```python
from build123d import *

# Parameters (mm, degrees)
BOSS_EXTRUDE1_DEPTH          = 90
SKETCH2_R                    = 7.55
SKETCH2_R_2                  = 5.5
CUT_EXTRUDE1_DEPTH           = 90
SKETCH3_R                    = 4.075
CUT_EXTRUDE2_DEPTH           = 90
CUT_EXTRUDE3_START           = -42
SKETCH4_W                    = 84
SKETCH4_H                    = 50
SKETCH4_R                    = 4.075
CUT_EXTRUDE3_DEPTH           = 42
SKETCH5_R                    = 11.5
SKETCH5_R_2                  = 1.75
CUT_EXTRUDE4_DEPTH           = 42
SKETCH10_W                   = 1
SKETCH10_H                   = 23.85052841
CUT_EXTRUDE_THIN1_DEPTH      = 70
CHAMFER2_SIZE                = 2
BOSS_EXTRUDE4_DEPTH          = 3
SKETCH15_W                   = 15
SKETCH15_H                   = 60
BOSS_EXTRUDE5_DEPTH          = 3
FILLET1_R                    = 5
SKETCH16_W                   = 84
SKETCH16_H                   = 42
CUT_EXTRUDE5_DEPTH           = 10
BOSS_EXTRUDE6_DEPTH          = 84
BOSS_EXTRUDE7_START          = -9
SKETCH18_R                   = 4.075
BOSS_EXTRUDE7_DEPTH          = 9
CUT_EXTRUDE_THIN3_DEPTH      = 121.933866311
CUT_EXTRUDE_THIN3_DEPTH_BACK = 9
SKETCH21_R                   = 11.5
CUT_EXTRUDE7_DEPTH           = 7
SKETCH22_R                   = 1.95
CUT_EXTRUDE8_DEPTH           = 20
SKETCH23_W                   = 15
SKETCH23_H                   = 5
CUT_EXTRUDE9_DEPTH           = 20
BOSS_EXTRUDE8_REACH          = 103.367
CHAMFER3_SIZE                = 5
CHAMFER4_SIZE                = 5


with BuildPart() as part:
    # Sketch1 → Boss-Extrude1 (new body)
    with BuildSketch(Plane(origin=(0, 0, 0), x_dir=(0, 0, -1), z_dir=(1, 0, 0))):
        with BuildLine():
            Line((-27.5, -30), (27.5, -30))
            ThreePointArc((27.5, -30), (31.035533906, -28.535533906), (32.5, -25))
            Line((32.5, -25), (32.5, 25))
            ThreePointArc((32.5, 25), (31.035533906, 28.535533906), (27.5, 30))
            Line((27.5, 30), (-27.5, 30))
            ThreePointArc((-27.5, 30), (-31.035533906, 28.535533906), (-32.5, 25))
            Line((-32.5, 25), (-32.5, -25))
            ThreePointArc((-32.5, -25), (-31.035533906, -28.535533906), (-27.5, -30))
        make_face()
    extrude(amount=BOSS_EXTRUDE1_DEPTH)

    # Sketch2 → Cut-Extrude1 (cut)
    with BuildSketch(Plane(origin=(0, 30, 0), x_dir=(1, 0, 0), z_dir=(0, 1, 0))):
        with Locations(Location((10, -18.5, 0), (0, 0, 270))):
            Circle(SKETCH2_R)
        with Locations(Location((80, -18.5, 0), (0, 0, 270))):
            Circle(SKETCH2_R)
        with Locations(Location((45, -18.5, 0), (0, 0, 270))):
            Circle(SKETCH2_R_2)
    extrude(amount=-CUT_EXTRUDE1_DEPTH, mode=Mode.SUBTRACT)

    # Sketch3 → Cut-Extrude2 (cut)
    with BuildSketch(Plane.XY.offset(32.5)):
        with Locations((20, 0)):
            Circle(SKETCH3_R)
        with Locations((70, 0)):
            Circle(SKETCH3_R)
    extrude(amount=-CUT_EXTRUDE2_DEPTH, mode=Mode.SUBTRACT)

    # Sketch4 → Cut-Extrude3 (cut)
    with BuildSketch(Plane(origin=(0, 0, -32.5), x_dir=(-1, 0, 0), z_dir=(0, 0, -1)).offset(CUT_EXTRUDE3_START)):
        with Locations((-45, 0)):
            Rectangle(SKETCH4_W, SKETCH4_H)
        with Locations(Location((-70, 0, 0), (0, 0, 180))):
            Circle(SKETCH4_R, mode=Mode.SUBTRACT)
        with Locations(Location((-20, 0, 0), (0, 0, 180))):
            Circle(SKETCH4_R, mode=Mode.SUBTRACT)
    extrude(amount=CUT_EXTRUDE3_DEPTH, mode=Mode.SUBTRACT)

    # Sketch5 → Cut-Extrude4 (cut)
    with BuildSketch(Plane(origin=(3, 0, 0), x_dir=(0, 0, -1), z_dir=(1, 0, 0))):
        with Locations((12, 0)):
            Circle(SKETCH5_R)
        with Locations((-3.5, 15.5)):
            Circle(SKETCH5_R_2)
        with Locations((27.5, 15.5)):
            Circle(SKETCH5_R_2)
        with Locations((27.5, -15.5)):
            Circle(SKETCH5_R_2)
        with Locations((-3.5, -15.5)):
            Circle(SKETCH5_R_2)
    extrude(amount=-CUT_EXTRUDE4_DEPTH, mode=Mode.SUBTRACT)

    # Sketch10 → Cut-Extrude-Thin1 (cut)
    with BuildSketch(Plane(origin=(0, 30, 0), x_dir=(1, 0, 0), z_dir=(0, 1, 0))):
        with Locations((10, -30.425264205)):
            Rectangle(SKETCH10_W, SKETCH10_H)
        with Locations((80, -30.425264205)):
            Rectangle(SKETCH10_W, SKETCH10_H)
    extrude(amount=-CUT_EXTRUDE_THIN1_DEPTH, mode=Mode.SUBTRACT)

    # Chamfer2
    chamfer2_edges = [part.edges().sort_by_distance(p)[0] for p in [
        (3, 0, -0.5),
    ]]
    chamfer(chamfer2_edges, length=CHAMFER2_SIZE)

    # Sketch14 → Boss-Extrude4 (add)
    with BuildSketch(Plane.ZY):
        with BuildLine():
            Line((-27.5, -30), (-42.5, -30))
            Line((-42.5, -30), (-42.5, 30))
            Line((-42.5, 30), (-27.5, 30))
            ThreePointArc((-27.5, 30), (-31.035533906, 28.535533906), (-32.5, 25))
            Line((-32.5, 25), (-32.5, -25))
            ThreePointArc((-32.5, -25), (-31.035533906, -28.535533906), (-27.5, -30))
        make_face()
    extrude(amount=-BOSS_EXTRUDE4_DEPTH)

    # Sketch15 → Boss-Extrude5 (add)
    with BuildSketch(Plane(origin=(90, 0, 0), x_dir=(0, 0, -1), z_dir=(1, 0, 0))):
        with Locations((35, 0)):
            Rectangle(SKETCH15_W, SKETCH15_H)
    extrude(amount=-BOSS_EXTRUDE5_DEPTH)

    # Fillet1
    fillet1_edges = [part.edges().sort_by_distance(p)[0] for p in [
        (1.5, -30, -42.5),
        (1.5, 30, -42.5),
        (88.5, 30, -42.5),
        (88.5, -30, -42.5),
    ]]
    fillet(fillet1_edges, radius=FILLET1_R)

    # Sketch16 → Cut-Extrude5 (cut)
    with BuildSketch(Plane(origin=(0, -25, 0), x_dir=(1, 0, 0), z_dir=(0, 1, 0))):
        with Locations((45, 11.5)):
            Rectangle(SKETCH16_W, SKETCH16_H)
    extrude(amount=-CUT_EXTRUDE5_DEPTH, mode=Mode.SUBTRACT)

    # Sketch17 → Boss-Extrude6 (add)
    with BuildSketch(Plane(origin=(3, 0, 0), x_dir=(0, 0, -1), z_dir=(1, 0, 0))):
        with BuildLine():
            Line((32.5, 25), (42.5, 25))
            ThreePointArc((42.5, 25), (41.035533906, 28.535533906), (37.5, 30))
            Line((37.5, 30), (27.5, 30))
            ThreePointArc((27.5, 30), (31.035533906, 28.535533906), (32.5, 25))
        make_face()
    extrude(amount=BOSS_EXTRUDE6_DEPTH)

    # Sketch18 → Boss-Extrude7 (add)
    with BuildSketch(Plane(origin=(0, 0, -42.5), x_dir=(-1, 0, 0), z_dir=(0, 0, -1)).offset(BOSS_EXTRUDE7_START)):
        with BuildLine():
            Line((-61, 0), (-61, 25))
            Line((-61, 25), (-87, 25))
            Line((-87, 25), (-87, -9))
            Line((-87, -9), (-70, -9))
            ThreePointArc((-70, -9), (-63.636038969, -6.363961031), (-61, 0))
        make_face()
        with Locations(Location((-70, 0, 0), (0, 0, 180))):
            Circle(SKETCH18_R, mode=Mode.SUBTRACT)
    extrude(amount=BOSS_EXTRUDE7_DEPTH)

    # Sketch19 → Cut-Extrude-Thin3 (cut, two sides: drawn at the far end of the back side and taken through both)
    with BuildSketch(Plane(origin=(0, 0, -42.5), x_dir=(-1, 0, 0), z_dir=(0, 0, -1)).offset(-CUT_EXTRUDE_THIN3_DEPTH_BACK)):
        Polygon((-61.965111244, -7.327781975), (-63.282485579, -6.01040764), (-66.764986476, -2.527906743), (-68.355005201, -0.937888018), (-69.062111982, -1.644994799), (-67.472093257, -3.235013524), (-63.98959236, -6.717514421), (-62.672218025, -8.034888756), align=None)
    extrude(amount=CUT_EXTRUDE_THIN3_DEPTH + CUT_EXTRUDE_THIN3_DEPTH_BACK, mode=Mode.SUBTRACT)

    # Sketch21 → Cut-Extrude7 (cut)
    with BuildSketch(Plane(origin=(0, 30, 0), x_dir=(1, 0, 0), z_dir=(0, 1, 0))):
        with Locations(Location((45, -18.5, 0), (0, 0, 231.500049591))):
            Circle(SKETCH21_R)
    extrude(amount=-CUT_EXTRUDE7_DEPTH, mode=Mode.SUBTRACT)

    # Sketch22 → Cut-Extrude8 (cut)
    with BuildSketch(Plane(origin=(0, 23, 0), x_dir=(1, 0, 0), z_dir=(0, 1, 0))):
        with Locations(Location((53, -18.5, 0), (0, 0, 270))):
            Circle(SKETCH22_R)
        with Locations(Location((45, -26.5, 0), (0, 0, 270))):
            Circle(SKETCH22_R)
        with Locations(Location((37, -18.5, 0), (0, 0, 270))):
            Circle(SKETCH22_R)
    extrude(amount=-CUT_EXTRUDE8_DEPTH, mode=Mode.SUBTRACT)

    # Sketch23 → Cut-Extrude9 (cut)
    with BuildSketch(Plane(origin=(3, 0, 0), x_dir=(0, 0, -1), z_dir=(1, 0, 0))):
        with Locations((12, 22.5)):
            Rectangle(SKETCH23_W, SKETCH23_H)
    extrude(amount=-CUT_EXTRUDE9_DEPTH, mode=Mode.SUBTRACT)

    # Sketch24 → Boss-Extrude8 (add, up to next)
    with BuildSketch(Plane.ZY.offset(-87), mode=Mode.PRIVATE) as boss_extrude8_sk1:
        with BuildLine():
            Line((-42.5, -21), (-33.5, -21))
            Line((-33.5, -21), (-33.5, -30))
            Line((-33.5, -30), (-37.5, -30))
            ThreePointArc((-37.5, -30), (-41.035533906, -28.535533906), (-42.5, -25))
            Line((-42.5, -25), (-42.5, -21))
        make_face()
    boss_extrude8_tool1 = extrude(boss_extrude8_sk1.sketch, amount=BOSS_EXTRUDE8_REACH, mode=Mode.PRIVATE) - part.part
    add(boss_extrude8_tool1.solids().sort_by_distance((87, -25.260021, -37.760021))[0])

    # Chamfer3
    chamfer3_edges = [part.edges().sort_by_distance(p)[0] for p in [
        (87, -9, -38),
        (3, -21, -38),
        (87, -21, -38),
    ]]
    chamfer(chamfer3_edges, length=CHAMFER3_SIZE)

    # Chamfer4
    # the kernel refuses this chamfer: 5 mm, written as the material it adds along each edge
    with BuildSketch(Plane(origin=(61, 25, -33.5), x_dir=(0.027495876610586317, -0.9996219169112968, 0), z_dir=(0, 0, -1))) as chamfer4_piece_1:
        Polygon((CHAMFER4_SIZE * 0.999621916911, CHAMFER4_SIZE * 0.0274958766106), (-CHAMFER4_SIZE * 0.0274958766106, CHAMFER4_SIZE * 0.999621916911), (0, 0), align=None)
    extrude(amount=9)


solid = part.part
```
The listing builds one solid part. Answer for the finished solid, in the listing's coordinates (mm). A direction names the side the tool comes from. Give positions to 0.01 mm unless a question says otherwise; leave off trailing zeros. Loops run counter-clockwise (first coordinate to the right, second up) from the corner with the lowest first, then second, coordinate; pieces in that order, holes last. Notation, with made-up numbers: M 78,33.25 L 119,33.25 A11 ccw 119,39.25 Z; hole C 47,-15 d5. An arc over 180 degrees is marked long. One line per item, written item: value.
Q1. For faces 1 (the face through (2, 22, -19.5)), 2 (the face through (85, -12, -38)), 3 (the face through (35.813, 13.14, 16.953)), determine the directions among +Z, -Z, +X, -X, +Y, -Y from which every point of the face is accessible in a straight line to the end or side of a thin tool.
Working result:
face 1: -X
face 2: -Z
face 3: +Y
Q2. A cutting plane is placed at A-A on y = 15.5. Give the number of separate pieces and of enclosed holes in the cut face, then the cut area to 3 significant figures.
Working result:
separate pieces: 3
enclosed holes: 4
area: 2,090 mm^2
Q3. Find the intervals of material crossed by line 1 (Y direction, x = 70, z = -37.75) (3 decimals); line 2 (X direction, y = 25, z = 18); line 3 (X direction, y = 7, z = -37.5), in increasing order. Write a range as from..to.
Working result:
line 1: y = -29.994..-21, -9..-4.075, 4.075..29.994
line 2: x = 0..2.47, 17.53..33.51, 56.49..72.47, 87.53..90
line 3: x = 0..3, 61..90
Q4. A cutting plane is placed at B-B on z = -27.5. Determine the outline of the cut face in (x, y), then the cut area to 3 significant figures.
Working result:
outline: M 0,-30 L 3,-30 L 3,-17.25 L 0,-17.25 Z; M 0,-13.75 L 3,-13.75 L 3,13.75 L 0,13.75 Z; M 0,17.25 L 3,17.25 L 3,25 L 87,25 L 87,-30 L 90,-30 L 90,30 L 0,30 Z
area: 759 mm^2
Q5. A cutting plane is placed at C-C on y = -23.5. Determine the outline of the cut face in (x, z).
Working result:
outline: M 0,-42.5 L 90,-42.5 L 90,32.5 L 80.5,32.5 L 80.5,26.03 A7.55 cw long 79.5,26.03 L 79.5,32.5 L 10.5,32.5 L 10.5,26.03 A7.55 cw long 9.5,26.03 L 9.5,32.5 L 0,32.5 Z; hole M 3,-33.5 L 87,-33.5 L 87,9.5 L 3,9.5 Z; hole C 45,18.5 d11
Q6. Flat-ended cylindrical pins translate along their axes: P1, Ø4.5, axis at x = 46, z = 26.5, coming from the +Y side; P2, Ø1.5, axis at y = -3.5, z = -8.5, coming from the -X side. Find the tip coordinate at first contact, or state that the pin passes through.
Working result:
P1: stops at y = 23
P2: stops at x = 87
Q7. A cutting plane is placed at D-D on x = 45. Determine the outline of the cut face in (y, z).
Working result:
outline: M -30,-37.5 A5 ccw -25,-42.5 L -21,-42.5 L -21,-33.5 L -30,-33.5 Z; M -30,9.5 L 23,9.5 L 23,13 L -30,13 Z; M -30,24 L 23,24 L 23,24.55 L 3,24.55 L 3,28.45 L 23,28.45 L 23,30 L 29.33,30 A5 ccw 25,32.5 L -25,32.5 A5 ccw -30,27.5 Z; M 25,-42.5 A5 ccw 30,-37.5 L 30,7 L 25,7 Z
Q8. Determine the mould class of faces 4 (the face through (44, -2, 9.5)), 5 (the face through (65.015, -4.278, -37.937)), 6 (the face through (4.68, -28.5, 31.07)) for opening direction Z: +Z half, -Z half, draft (parallel to the pull), parting line (faces both ways), or undercut.
Working result:
face 4: undercut
face 5: draft
face 6: +Z half
